Autodesk Inventor part; units mm, degrees
ref_plane "YZ Plane" through (0, 0, 0) normal (1, 0, 0) x (0, 1, 0)
ref_plane "XZ Plane" through (0, 0, 0) normal (0, 1, 0) x (-1, 0, 0)
ref_plane "XY Plane" through (0, 0, 0) normal (0, 0, 1) x (1, 0, 0)
sketch3d "3D Sketch1"
sketch "Sketch8" plane through (0, 0, 0) normal (0, 1, 0) x (-1, 0, 0)
  arc A0 (-533.9727, 129.2939) -> (-533.9727, 72.7061) centre (-524, 101) ccw
  arc A1 (-533.9727, 129.2939) -> (-540.6211, 148.1565) centre (-537.2969, 138.7252) ccw
  arc A2 (-540.6211, 148.1565) -> (-540.6211, 53.8435) centre (-524, 101) ccw
  arc A3 (-540.6211, 53.8435) -> (-533.9727, 72.7061) centre (-537.2969, 63.2748) ccw
  circle A4 centre (-537.2969, 63.2748) radius 3
  circle A5 centre (-556.6482, 77.8001) radius 2.9994
  circle A6 centre (-564, 101) radius 3
  circle A7 centre (-556.6482, 124.1094) radius 2.9994
  circle A8 centre (-537.2969, 138.7252) radius 3
  line L0 (-531, 98.5) -> (-531, 115.5)
  line L1 (-451.3425, 101.8066) -> (-466.8633, 88.0104)
  arc A9 (-451.3425, 101.8066) -> (-450, 104.7963) centre (-454, 104.7963) ccw
  line L2 (-450, 109.2037) -> (-450, 104.7963)
  arc A10 (-450, 109.2037) -> (-451.3425, 112.1934) centre (-454, 109.2037) ccw
  line L3 (-466.8633, 125.9896) -> (-451.3425, 112.1934)
  arc A11 (-466.8633, 125.9896) -> (-469.5208, 127) centre (-469.5208, 123) ccw
  line L4 (-505.0775, 127) -> (-469.5208, 127)
  arc A12 (-505.0775, 127) -> (-508.201, 125.4988) centre (-505.0775, 123) ccw
  line L5 (-511.799, 121.0012) -> (-508.201, 125.4988)
  arc A13 (-514.9225, 119.5) -> (-511.799, 121.0012) centre (-514.9225, 123.5) ccw
  line L6 (-527, 119.5) -> (-514.9225, 119.5)
  arc A14 (-527, 119.5) -> (-531, 115.5) centre (-527, 115.5) ccw
  arc A15 (-531, 98.5) -> (-527, 94.5) centre (-527, 98.5) ccw
  line L7 (-514.9225, 94.5) -> (-527, 94.5)
  arc A16 (-511.799, 92.9988) -> (-514.9225, 94.5) centre (-514.9225, 90.5) ccw
  line L8 (-508.201, 88.5012) -> (-511.799, 92.9988)
  arc A17 (-508.201, 88.5012) -> (-505.0775, 87) centre (-505.0775, 91) ccw
  line L9 (-469.5208, 87) -> (-505.0775, 87)
  line L10 (-478, 91.45) -> (-470, 91.45)
  arc A18 (-470, 91.45) -> (-470, 94.55) centre (-470, 93) ccw
  line L11 (-470, 94.55) -> (-478, 94.55)
  arc A19 (-478, 94.55) -> (-478, 91.45) centre (-478, 93) ccw
  arc A20 (-495, 91.45) -> (-495, 94.55) centre (-495, 93) ccw
  line L12 (-503, 91.45) -> (-495, 91.45)
  arc A21 (-503, 94.55) -> (-503, 91.45) centre (-503, 93) ccw
  line L13 (-495, 94.55) -> (-503, 94.55)
  line L14 (-455, 105.5) -> (-469, 105.5)
  arc A22 (-455, 105.5) -> (-455, 108.5) centre (-455, 107) ccw
  line L15 (-469, 108.5) -> (-455, 108.5)
  arc A23 (-469, 108.5) -> (-469, 105.5) centre (-469, 107) ccw
  arc A24 (-482, 105.45) -> (-482, 108.55) centre (-482, 107) ccw
  line L16 (-490, 105.45) -> (-482, 105.45)
  arc A25 (-490, 108.55) -> (-490, 105.45) centre (-490, 107) ccw
  line L17 (-482, 108.55) -> (-490, 108.55)
  line L18 (-501, 109) -> (-501, 105)
  line L19 (-501, 105) -> (-511, 105)
  line L20 (-511, 105) -> (-511, 109)
  line L21 (-511, 109) -> (-501, 109)
  circle A26 centre (-525.75, 100) radius 1.55
  circle A27 centre (-525.75, 114) radius 1.55
  arc A28 (-503, 122.55) -> (-503, 119.45) centre (-503, 121) ccw
  line L22 (-503, 122.55) -> (-495, 122.55)
  arc A29 (-495, 119.45) -> (-495, 122.55) centre (-495, 121) ccw
  line L23 (-495, 119.45) -> (-503, 119.45)
  arc A30 (-478, 122.55) -> (-478, 119.45) centre (-478, 121) ccw
  line L24 (-478, 122.55) -> (-470, 122.55)
  arc A31 (-470, 119.45) -> (-470, 122.55) centre (-470, 121) ccw
  line L25 (-470, 119.45) -> (-478, 119.45)
  arc A32 (-469.5208, 87) -> (-466.8633, 88.0104) centre (-469.5208, 91) ccw
  line L26 (-487, 7.43) -> (-478.1, 7.43)
  line L27 (-495.9, 7.43) -> (-487, 7.43)
  arc A33 (-495.9, 7.43) -> (-499.5, 3.83) centre (-495.9, 3.83) ccw
  line L28 (-499.5, -0.5942) -> (-499.5, 3.83)
  arc A34 (-499.5, -0.5942) -> (-498.1907, -3.5539) centre (-495.5, -0.5942) ccw
  line L29 (-490, -11) -> (-498.1907, -3.5539)
  line L30 (-484, -11) -> (-490, -11)
  line L31 (-475.8093, -3.5539) -> (-484, -11)
  arc A35 (-475.8093, -3.5539) -> (-474.5, -0.5942) centre (-478.5, -0.5942) ccw
  line L32 (-474.5, 3.83) -> (-474.5, -0.5942)
  arc A36 (-474.5, 3.83) -> (-478.1, 7.43) centre (-478.1, 3.83) ccw
  arc A37 (-478.45, 4) -> (-481.55, 4) centre (-480, 4) ccw
  line L33 (-481.55, 4) -> (-481.55, -1)
  arc A38 (-481.55, -1) -> (-478.45, -1) centre (-480, -1) ccw
  line L34 (-478.45, -1) -> (-478.45, 4)
  line L35 (-492.45, 4) -> (-492.45, -1)
  arc A39 (-492.45, 4) -> (-495.55, 4) centre (-494, 4) ccw
  line L36 (-495.55, -1) -> (-495.55, 4)
  arc A40 (-495.55, -1) -> (-492.45, -1) centre (-494, -1) ccw
  arc A41 (-494.09, 79.2321) -> (-479.91, 79.2321) centre (-487, 84) ccw
  arc A42 (-494.09, 79.2321) -> (-497.4092, 81) centre (-497.4092, 77) ccw
  line L37 (-497.4092, 81) -> (-503, 81)
  arc A43 (-503, 81) -> (-507, 77) centre (-503, 77) ccw
  line L38 (-507, 77) -> (-507, 50.7937)
  arc A44 (-511.1379, 43.7877) -> (-507, 50.7937) centre (-515, 50.7937) ccw
  arc A45 (-511.1379, 43.7877) -> (-462.8621, 43.7877) centre (-487, 0) ccw
  arc A46 (-467, 50.7937) -> (-462.8621, 43.7877) centre (-459, 50.7937) ccw
  line L39 (-467, 50.7937) -> (-467, 77)
  arc A47 (-467, 77) -> (-471, 81) centre (-471, 77) ccw
  line L40 (-471, 81) -> (-476.5908, 81)
  arc A48 (-476.5908, 81) -> (-479.91, 79.2321) centre (-476.5908, 77) ccw
  circle A49 centre (-473, 75) radius 1.25
  circle A50 centre (-501, 75) radius 1.25
  circle A51 centre (-487, 63) radius 1.25
  circle A52 centre (-470.7, 62.6926) radius 1.25
  circle A53 centre (-473, 50) radius 1.25
  circle A54 centre (-501, 50) radius 1.25
  circle A55 centre (-470.7, 37.4926) radius 1.25
  arc A56 (-485, 53) -> (-489, 53) centre (-487, 53) ccw
  line L41 (-485, 37) -> (-485, 53)
  line L42 (-489, 53) -> (-489, 37)
  arc A57 (-489, 37) -> (-485, 37) centre (-487, 37) ccw
  arc A58 (-513.2873, 34.029) -> (-460.7127, 34.0291) centre (-487, 0) ccw
  arc A59 (-509.6193, 29.2808) -> (-464.3807, 29.2808) centre (-487, 0) ccw
  arc A60 (-460.7127, 34.0291) -> (-464.3807, 29.2808) centre (-462.5467, 31.6549) ccw
  arc A61 (-509.6193, 29.2808) -> (-513.2873, 34.029) centre (-511.4533, 31.6549) ccw
  arc A62 (-496, 32) -> (-500, 28) centre (-496, 28) ccw
  line L43 (-496, 32) -> (-478, 32)
  arc A63 (-474, 28) -> (-478, 32) centre (-478, 28) ccw
  line L44 (-474, 28) -> (-474, 22)
  arc A64 (-474, 22) -> (-470, 18) centre (-470, 22) ccw
  line L45 (-470, 18) -> (-465.0911, 18)
  arc A65 (-461.7205, 16.1538) -> (-465.0911, 18) centre (-465.0911, 14) ccw
  arc A66 (-512.2795, 16.1538) -> (-461.7205, 16.1538) centre (-487, 0) ccw
  arc A67 (-508.9089, 18) -> (-512.2795, 16.1538) centre (-508.9089, 14) ccw
  line L46 (-508.9089, 18) -> (-504, 18)
  arc A68 (-504, 18) -> (-500, 22) centre (-504, 22) ccw
  line L47 (-500, 22) -> (-500, 28)
  point P0 (0, 0)
extrude "Extrusion1" add sketch "Sketch8" along normal blind 3 contours A41 A48 L40 A47 L39 A46 A45 A44 L38 A43 L37 A42
properties part number "pulsador_monta_riel"
Could you check a few things on this model? Use its own coordinates, in mm. A direction names the side the tool comes from. Round coordinates to 2 decimals unless told otherwise and drop trailing zeros. Write each loop counter-clockwise with the first axis right and the second up, starting at its lowest first coordinate (ties: lowest second). Pieces come first, ordered by that corner, then holes. Notation, with made-up numbers: (80.5, 25) - (94.5, 25) arc R10 ccw to (94.5, 35) - close; hole circle Ø4 at (-40, 79). An arc over 180 degrees is marked (long way). Use a Markdown table: item, result.
Q1. For pin 1 (0.9 mm diameter, centred on y = 2, z = 70.5, fed in from -X); pin 2 (0.9 mm diameter, centred on x = 467, y = 2, fed in from -Z); pin 3 (1.5 mm diameter, centred on x = 483.5, y = 1.5, fed in from -Z); pin 4 (3 mm diameter, centred on x = 470.7, z = 37.49, fed in from -Y), each with a flat end and sliding along its axis, tell me the tip position at first contact or that it passes through.
Output values:
| item | result |
|---|---|
| pin 1 | x = 467 |
| pin 2 | z = -46.02 |
| pin 3 | z = -49.92 |
| pin 4 | y = 0 |
Q2. Thinking about a two-plate mould opening in Z: for faces 1 (the cylindrical face through (486.883, 1.479, 75.457)), 2 (the flat face through (500, 1, 25)), 3 (the cylindrical face through (470.028, 1.479, 36.439)), 4 (the cylindrical face through (485.154, 1.479, -49.966)), which applies, released by +Z, released by -Z, zero draft, split by the parting line, or undercut?
Output values:
| item | result |
|---|---|
| face 1 | released by +Z |
| face 2 | undercut |
| face 3 | undercut |
| face 4 | split by the parting line |
Q3. I want a section at A-A (x = 518.5). List the corners of the cut face in (y, z) for me, plus the area to 3 significant figures.
Output values:
| item | result |
|---|---|
| outline | (0, -38.83) - (3, -38.83) - (3, -29.27) - (0, -29.27) - close; (0, -19.41) - (3, -19.41) - (3, 19.41) - (0, 19.41) - close; (0, 29.27) - (3, 29.27) - (3, 38.83) - (0, 38.83) - close |
| area | 174 mm2 |
Q4. Please list where these lines run through material, in increasing order: L1, parallel to X at y = 2.1, z = 75; L2, parallel to Z at x = 501, y = 2.1; L3, parallel to X at y = 2.35, z = 0.
Output values:
| item | result |
|---|---|
| L1 | 467 to 471.75, 474.25 to 499.75, 502.25 to 507 |
| L2 | -48 to -40.66, -34.25 to -26.53, 19.35 to 48.75, 51.25 to 73.75, 76.25 to 81 |
| L3 | 437 to 444, 450 to 457, 517 to 524, 530 to 537 |
Q5. I want a section at D-D (z = -16.5). List the corners of the cut face in (x, y) for me.
Output values:
| item | result |
|---|---|
| outline | (439.8, 0) - (447.29, 0) - (447.29, 3) - (439.8, 3) - close; (453.88, 0) - (461.95, 0) - (461.95, 3) - (453.88, 3) - close; (512.05, 0) - (520.12, 0) - (520.12, 3) - (512.05, 3) - close; (526.71, 0) - (534.2, 0) - (534.2, 3) - (526.71, 3) - close |
Q6. I want a section at B-B (z = -35.5). List the corners of the cut face in (x, y) for me.
Output values:
| item | result |
|---|---|
| outline | (451.79, 0) - (462.74, 0) - (462.74, 3) - (451.79, 3) - close; (476.57, 0) - (497.43, 0) - (497.43, 3) - (476.57, 3) - close; (511.26, 0) - (522.21, 0) - (522.21, 3) - (511.26, 3) - close |
Q7. I want a section at C-C (z = 20). List the corners of the cut face in (x, y) for me, plus the area to 3 significant figures.
Output values:
| item | result |
|---|---|
| outline | (441.17, 0) - (448.93, 0) - (448.93, 3) - (441.17, 3) - close; (455.87, 0) - (473.46, 0) - (473.46, 3) - (455.87, 3) - close; (500.54, 0) - (518.13, 0) - (518.13, 3) - (500.54, 3) - close; (525.07, 0) - (532.83, 0) - (532.83, 3) - (525.07, 3) - close |
| area | 152 mm2 |
Q8. For faces 5 (the cylindrical face through (495.55, 1.48, 80.54)), 6 (the cylindrical face through (508.08, 1.48, 46.78)), 7 (the flat face through (467, 1, 64)), 8 (the cylindrical face through (472.797, 1.479, 19.141)), which set-ups out of +Z, -Z, +X, -X, +Y, -Y let a thin tool reach every point of the face, with its end or its side?
Output values:
| item | result |
|---|---|
| face 5 | +Z, +Y, -Y |
| face 6 | +Z, +X, +Y, -Y |
| face 7 | +Z, -X, +Y, -Y |
| face 8 | +Y, -Y |
